from build123d import *

# Parameters (mm, degrees)
SKETCH_1_R          = 10
EXTRUDE_1_DEPTH     = 16.4
SKETCH_2_R          = 8.85
CUT_EXTRUDE_1_DEPTH = 0.7
SKETCH_3_R          = 1.325
EXTRUDE_2_DEPTH     = 5
CHAMFER_1_SIZE      = 0.8
SKETCH_4_R          = 8.05
CUT_EXTRUDE_2_DEPTH = 0.4
FILLET_1_R          = 0.8
SKETCH_5_R          = 7
EXTRUDE_3_DEPTH     = 0.2


with BuildPart() as part:
    # Эскиз1 → Бобышка-Вытянуть1 (new body)
    with BuildSketch(Plane.XY):
        Circle(SKETCH_1_R)
    extrude(amount=EXTRUDE_1_DEPTH)

    # Эскиз2 → Вырез-Вытянуть1 (cut)
    with BuildSketch(Plane.XY.offset(16.4)):
        Circle(SKETCH_2_R)
    extrude(amount=-CUT_EXTRUDE_1_DEPTH, mode=Mode.SUBTRACT)

    # Эскиз3 → Бобышка-Вытянуть2 (add)
    with BuildSketch(Plane.XY.offset(15.7)):
        with Locations((-4.775, 4.775)):
            Circle(SKETCH_3_R)
        with Locations((-4.775, -4.775)):
            Circle(SKETCH_3_R)
        with Locations((4.775, 4.775)):
            Circle(SKETCH_3_R)
    extrude(amount=EXTRUDE_2_DEPTH)

    # Фаска1
    chamfer_1_edges = [part.edges().sort_by_distance(p)[0] for p in [
        (-6.1, 4.775, 20.7),
        (-6.1, -4.775, 20.7),
        (3.45, 4.775, 20.7),
    ]]
    chamfer(chamfer_1_edges, length=CHAMFER_1_SIZE)

    # Эскиз4 → Вырез-Вытянуть2 (cut)
    with BuildSketch(Plane(origin=(0, 0, 0), x_dir=(-1, 0, 0), z_dir=(0, 0, -1))):
        Circle(SKETCH_4_R)
    extrude(amount=-CUT_EXTRUDE_2_DEPTH, mode=Mode.SUBTRACT)

    # Скругление1
    fillet_1_edges = [part.edges().sort_by_distance(p)[0] for p in [
        (-10, 0, 0),
        (-10, 0, 16.4),
    ]]
    fillet(fillet_1_edges, radius=FILLET_1_R)

    # Эскиз5 → Бобышка-Вытянуть3 (add)
    with BuildSketch(Plane(origin=(0, 0, 0.4), x_dir=(-1, 0, 0), z_dir=(0, 0, -1))):
        Circle(SKETCH_5_R)
    extrude(amount=EXTRUDE_3_DEPTH)


solid = part.part
Verification items for the finished model (mm, model axes). A direction names the side the tool comes from. Round coordinates to 2 decimals unless told otherwise and drop trailing zeros. Order: outer loops, then holes, each group sorted by start corner. A loop starts at its lowest first (then second) coordinate and runs counter-clockwise, first axis right, second up.
1. Go/stop test with flat-tipped pins: P1, Ø1.5, axis at x = -3, y = 3, coming from the -Z side; P2, Ø5.5, axis at x = -1, y = 1, coming from the +Z side; P3, Ø4, axis at y = -4.5, z = 15, coming from the -X side. Record where each tip stops, or that it passes through.
Final values:
P1: stops at z = 0.2
P2: stops at z = 15.7
P3: stops at x = -9.68
2. Release check for a two-part mould opening along Y. For faces 4 (the flat face through (-5, -5, 20.7)), 5 (the cylindrical face through (-2.17, -9.76, 8.1)), 6 (the cylindrical face through (-7.678, 2.418, 0.197)) record: +Y half, -Y half, draft (parallel to the pull), parting line (faces both ways), or undercut.
Final values:
face 4: draft
face 5: parting line
face 6: undercut
3. Access from +Z, -Z, +X, -X, +Y, -Y to the whole of each face (thin tool, end or side, straight path). Record for faces 1 (the flat face through (3.4, -7.5, 0)), 2 (the cylindrical face through (4.6, 6.09, 17.77)), 3 (the flat face through (2, 7, 0.4)).
Final values:
face 1: -Z, +X, -X, +Y, -Y
face 2: +Z
face 3: -Z
4. Section check C-C on z = 9. Record the cut outline in (x, y), then the cut area to 3 significant figures.
Final values:
outline: circle Ø20 at (0, 0)
area: 314 mm2
5. Section check A-A on y = 0. Record the cut outline in (x, z).
Final values:
outline: (-10, 0.8) arc R0.8 ccw to (-9.2, 0) - (-8.05, 0) - (-8.05, 0.4) - (-7, 0.4) - (-7, 0.2) - (7, 0.2) - (7, 0.4) - (8.05, 0.4) - (8.05, 0) - (9.2, 0) arc R0.8 ccw to (10, 0.8) - (10, 15.6) arc R0.8 ccw to (9.2, 16.4) - (8.85, 16.4) - (8.85, 15.7) - (-8.85, 15.7) - (-8.85, 16.4) - (-9.2, 16.4) arc R0.8 ccw to (-10, 15.6) - close
6. Thickness scan on L1, parallel to Y at x = 0, z = 0.35; L2, parallel to X at y = -4.25, z = 16; L3, parallel to Z at x = 4, y = -2.5. Record the ranges inside material, lowest first.
Final values:
L1: y = -9.86 to -8.05, -7 to 7, 8.05 to 9.86
L2: x = -8.93 to -7.76, -5.99 to -3.56, 7.76 to 8.93
L3: z = 0.2 to 15.7
